Part model, mm, in its own coordinate system. A direction names the side the tool comes from. Coordinates: 2 decimals unless noted, no trailing zeros. Loops run counter-clockwise (first coordinate to the right, second up) from the corner with the lowest first, then second, coordinate; pieces in that order, holes last. Notation, with made-up numbers: (9, 21) -> (49, 21) arc R20 ccw to (49, 40) -> close; hole circle Ø2 at (6, 37). An arc over 180 degrees is marked (long way). One line per question, with ' | ' between items. Start each with the question number.
1) 3-axis set-ups, long thin cutter, end or side, ignore diameter. For faces 1 (the face through (-1.4, -1.7, -4)), 2 (the face through (0, -1.45, 3)), 3 (the face through (0.026, -3.135, -4.507)): which of +Z, -Z, +X, -X, +Y, -Y reach the whole face in a straight line?
2) Cut at A-A (z = 2). List the corners of the cut face in (x, y).
3) Two-plate mould, pull along X, no slides. Class faces 4 (the face through (0, -1, 0)), 5 (the face through (2.45, -2.43, -4.51)), 6 (the face through (-2.43, -2.45, -4.51)): released by +X, released by -X, zero draft, split by the parting line, or undercut.
4) Cut at C-C (x = 0). List the corners of the cut face in (y, z), plus the area to 3 significant figures.
5) Cut at B-B (y = 0). List the corners of the cut face in (x, z).
6) Probe L1, parallel to Y at x = 0, z = 2.5; L2, parallel to Y at x = 0, z = -2.5; L3, parallel to Z at x = 0, y = 1.5. List the from-to ranges inside material, lowest first. Write a range as from..to.
7) Cut at D-D (y = -1.25). List the corners of the cut face in (x, z).
8) Drop flat-ended pins along their axis: pin 1 (0.8 mm diameter, centred on x = -0.5, z = 2.5, fed in from +Y); pin 2 (1 mm diameter, centred on x = -2.5, y = -1, fed in from +Z); pin 3 (1.3 mm diameter, centred on x = -0.5, z = 2.5, fed in from -Y). Give the stop position or say it passes through.
from build123d import *

# Parameters (mm, degrees)
SKETCH_1_R          = 1.95
SKETCH_1_R_2        = 1
EXTRUDE_1_DEPTH     = 5
EXTRUDE_3_DEPTH     = 1
SKETCH_5_W          = 3.686325021
SKETCH_5_H          = 0.905885224
SKETCH_5_W_2        = 4.457672836
SKETCH_5_H_2        = 1.506818987
CUT_EXTRUDE_4_DEPTH = 4.5


with BuildPart() as part:
    # 草图1 → 凸台-拉伸1 (new body, symmetric)
    with BuildSketch(Plane.XY):
        Circle(SKETCH_1_R)
        Circle(SKETCH_1_R_2, mode=Mode.SUBTRACT)
    extrude(amount=EXTRUDE_1_DEPTH, both=True)

    # 草图3 → 凸台-拉伸3 (add)
    with BuildSketch(Plane(origin=(0, 0, -5), x_dir=(-1, 0, 0), z_dir=(0, 0, -1))):
        with BuildLine():
            ThreePointArc((-0.668047872, 3.384702652), (-2.447870462, 2.431137635), (-3.389205192, 0.644816382))
            ThreePointArc((-3.389205192, 0.644816382), (-3.838268125, -0.013163552), (-3.384702652, -0.668047872))
            ThreePointArc((-3.384702652, -0.668047872), (-2.431137635, -2.447870462), (-0.644816382, -3.389205192))
            ThreePointArc((-0.644816382, -3.389205192), (0.013163552, -3.838268125), (0.668047872, -3.384702652))
            ThreePointArc((0.668047872, -3.384702652), (2.447870462, -2.431137635), (3.389205192, -0.644816382))
            ThreePointArc((3.389205192, -0.644816382), (3.838268125, 0.013163552), (3.384702652, 0.668047872))
            ThreePointArc((3.384702652, 0.668047872), (2.431137635, 2.447870462), (0.644816382, 3.389205192))
            ThreePointArc((0.644816382, 3.389205192), (-0.013163552, 3.838268125), (-0.668047872, 3.384702652))
        make_face()
        with BuildLine():
            Line((2.551831088, 1.821511161), (1.580005505, 1.142839711))
            ThreePointArc((1.580005505, 1.142839711), (1.364402664, 1.393163799), (1.109636091, 1.603498596))
            Line((1.109636091, 1.603498596), (1.804122226, 2.564154403))
            ThreePointArc((1.804122226, 2.564154403), (0.024621795, 3.135145702), (-1.763627121, 2.592173641))
            Line((-1.763627121, 2.592173641), (-1.109636091, 1.603498596))
            ThreePointArc((-1.109636091, 1.603498596), (-1.383616658, 1.374083311), (-1.611132184, 1.098523138))
            Line((-1.611132184, 1.098523138), (-2.590192379, 1.766535663))
            ThreePointArc((-2.590192379, 1.766535663), (-3.135242384, 0), (-2.590192379, -1.766535663))
            Line((-2.590192379, -1.766535663), (-1.611132184, -1.098523138))
            ThreePointArc((-1.611132184, -1.098523138), (-1.383616658, -1.374083311), (-1.109636091, -1.603498596))
            Line((-1.109636091, -1.603498596), (-1.763627121, -2.592173641))
            ThreePointArc((-1.763627121, -2.592173641), (0, -3.135242384), (1.763627121, -2.592173641))
            Line((1.763627121, -2.592173641), (1.109636091, -1.603498596))
            ThreePointArc((1.109636091, -1.603498596), (1.383616658, -1.374083311), (1.611132184, -1.098523138))
            Line((1.611132184, -1.098523138), (2.590192379, -1.766535663))
            ThreePointArc((2.590192379, -1.766535663), (3.135063211, 0.033518256), (2.551831088, 1.821511161))
        make_face(mode=Mode.SUBTRACT)
    extrude(amount=-EXTRUDE_3_DEPTH)

    # 草图5 → 切除-拉伸4 (cut)
    with BuildSketch(Plane.XY.offset(5)):
        with Locations((-0.148639524, 1.902942612)):
            Rectangle(SKETCH_5_W, SKETCH_5_H)
        with Locations((0.156311938, -2.203409494)):
            Rectangle(SKETCH_5_W_2, SKETCH_5_H_2)
    extrude(amount=-CUT_EXTRUDE_4_DEPTH, mode=Mode.SUBTRACT)


solid = part.part
Reported:
1) face 1: +Z | face 2: +Z, +X, -X, -Y | face 3: +Z, -Z
2) outline: (-1.3, -1.45) -> (1.3, -1.45) arc R1.95 ccw to (1.3, 1.45) -> (-1.3, 1.45) arc R1.95 ccw to start; hole circle Ø2 at (0, 0)
3) face 4: undercut | face 5: released by +X | face 6: released by -X
4) outline: (-3.84, -5) -> (-3.14, -5) -> (-3.14, -4) -> (-3.84, -4) -> close; (-1.95, -5) -> (-1, -5) -> (-1, 5) -> (-1.45, 5) -> (-1.45, 0.5) -> (-1.95, 0.5) -> close; (1, -5) -> (1.95, -5) -> (1.95, 0.5) -> (1.45, 0.5) -> (1.45, 5) -> (1, 5) -> close; (3.14, -5) -> (3.84, -5) -> (3.84, -4) -> (3.14, -4) -> close | area: 15.9 mm²
5) outline: (-3.84, -5) -> (-3.14, -5) -> (-3.14, -4) -> (-3.84, -4) -> close; (-1.95, -5) -> (-1, -5) -> (-1, 5) -> (-1.95, 5) -> close; (1, -5) -> (1.95, -5) -> (1.95, 5) -> (1, 5) -> close; (3.14, -5) -> (3.84, -5) -> (3.84, -4) -> (3.14, -4) -> close
6) L1: y = -1.45..-1, 1..1.45 | L2: y = -1.95..-1, 1..1.95 | L3: z = -5..0.5
7) outline: (-3.22, -5) -> (-2.88, -5) -> (-2.88, -4) -> (-3.22, -4) -> close; (-1.83, -5) -> (1.83, -5) -> (1.83, -4) -> (1.5, -4) -> (1.5, 5) -> (-1.5, 5) -> (-1.5, -4) -> (-1.83, -4) -> close; (2.88, -5) -> (3.22, -5) -> (3.22, -4) -> (2.88, -4) -> close
8) pin 1: stops at y = 1.45 | pin 2: stops at z = -4 | pin 3: stops at y = -1.45
